Design review of the part built by this model. Coordinates are the model's own, in mm. Coordinates: 2 decimals unless noted, no trailing zeros. Write each loop counter-clockwise with the first axis right and the second up, starting at its lowest first coordinate (ties: lowest second). Pieces come first, ordered by that corner, then holes. Notation, with made-up numbers: M -19,84 L 2,84 A14 cw 2,89 Z; hole C 52.25,-21 d7. An arc over 180 degrees is marked long. One line per question, with ' | ' between items.
Autodesk Inventor part; units mm, degrees
ref_plane "Work Plane2" through (5, 0, 0) normal (0.2588, 0.9659, 0) x (-0.9659, 0.2588, 0)
ref_plane "YZ Plane" through (0, 0, 0) normal (1, 0, 0) x (0, 1, 0)
ref_plane "XZ Plane" through (0, 0, 0) normal (0, 1, 0) x (-1, 0, 0)
sketch "Sketch1" plane through (0, 0, 0) normal (0, 0, 1) x (1, 0, 0)
  line L0 (0, -0.2679) -> (0, 1.6077)
  line L1 (3.0681, 0) -> (5, 0)
  line L2 (5, 0) -> (0.3349, 1.25)
  line L3 (0, 1.3397) -> (0, 0)
  line L4 (0, 0) -> (0.3349, 1.25) construction
  line L5 (0, 0) -> (1.2941, 0) construction
  line L6 (0.3349, 1.25) -> (0.2055, 0.767)
  line L7 (0.2055, 0.767) -> (3.0681, 0)
  dimension "d2" = 5
  dimension "d3" = 15
  dimension "d4" = 75
  dimension "d16" = 0.5
revolve "Revolution1" add sketch "Sketch1" angle 360 about axis through (0, -10, 0) along (0, 1, 0)
ref_plane "Work Plane2" through (5, 0, 0) normal (0.2588, 0.9659, 0) x (-0.9659, 0.2588, 0)
sketch "Sketch5" plane through (5, 0, 0) normal (0.2588, 0.9659, 0) x (-0.9659, 0.2588, 0)
  circle A0 centre (2.7092, 0) radius 1
  point P0 (4.8296, 0)
  dimension "d18" = 2
extrude "Extrusion2" cut sketch "Sketch5" against normal through all
pattern_circular "Circular Pattern3" count 3 over 360 about axis through (0, -10, 0) along (0, 1, 0) of "Extrusion2"
properties part number "Splitter"
1. Take a section at A-A (z = 0). Write out the cut boundary in (x, y).
Answer sheet:
outline: M -5,0 L -3.07,0 L -0.21,0.77 L -0.33,1.25 Z; M 0.21,0.77 L 1.29,0.48 L 1.42,0.96 L 0.33,1.25 Z; M 3.23,0 L 5,0 L 3.35,0.44 Z
2. Take a section at B-B (x = 0). Write out the cut boundary in (y, z).
Answer sheet:
outline: M 0,-5 L 1.25,-0.33 L 0.77,-0.21 L 0,-3.07 Z; M 0,3.07 L 0.77,0.21 L 1.25,0.33 L 0,5 Z
3. Draft analysis for pull direction X (two halves, no side actions). For faces 1 (the face through (-0.1, 0, 3.3)), 2 (the face through (0.29, 1.17, -0.56)), 3 (the face through (1.42, 0.675, -0.383)), 4 (the face through (-0.956, 0.683, 1.054)), state which applies: pulls with the +X half, pulls with the -X half, needs draft (parallel to the pull), parting line crosses it, or undercut.
Answer sheet:
face 1: needs draft | face 2: parting line crosses it | face 3: undercut | face 4: undercut
4. Insertion check: pin 1 Ø2 at (x, z) = (2.5, -2) entering from -Y. The pin has a flat end and moves straight along its axis. Give the tip position at first contact, or say it passes through.
Answer sheet:
pin 1: y = 0
5. To check wall thickness, follow line 1 along Y through (x, z) = (-3.75, 0.25); line 2 along Y through (x, z) = (0.5, -2.75). State the ranges of each line that lie inside material, in increasing order. Write a range as [from, to].
Answer sheet:
line 1: [0, 0.33] | line 2: [0.07, 0.59]
